from build123d import *

# Parameters (mm, degrees)
SKETCH2_R           = 101.6
SKETCH2_R_2         = 76.2
BOSS_EXTRUDE1_DEPTH = 38.1
FILLET2_R           = 12.7
SHELL1_T            = -6.35


with BuildPart() as part:
    # Sketch2 → Boss-Extrude1 (new, symmetric)
    with BuildSketch(Plane.XY):
        with Locations(Location((0, 0, 0), (0, 0, 180))):
            Circle(SKETCH2_R)
        with Locations(Location((0, 0, 0), (0, 0, 180))):
            Circle(SKETCH2_R_2, mode=Mode.SUBTRACT)
    extrude(amount=BOSS_EXTRUDE1_DEPTH, both=True)

    # Fillet2
    fillet2_edges = [part.edges().sort_by_distance(p)[0] for p in [
        (101.6, 0, -38.1),
        (101.6, 0, 38.1),
    ]]
    fillet(fillet2_edges, radius=FILLET2_R)

    # Shell1
    shell1_openings = [part.faces().sort_by_distance(p)[0] for p in [
        (76.2, 0, 0),
    ]]
    offset(amount=SHELL1_T, openings=shell1_openings, kind=Kind.INTERSECTION)


solid = part.part
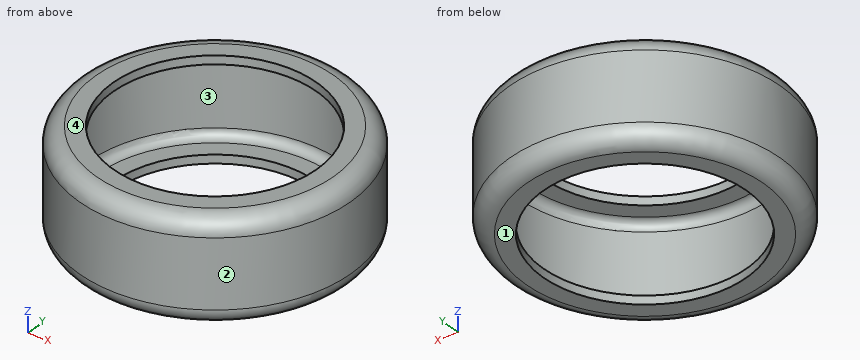
Here's how the part is built. I have some questions about the finished solid (model axes, mm). Face numbers are marked on the shaded views. Round coordinates to 2 decimals unless told otherwise and drop trailing zeros. Loops run counter-clockwise (first coordinate to the right, second up) from the corner with the lowest first, then second, coordinate; pieces in that order, holes last. Notation, with made-up numbers: (-10, -7) - (7, -7) arc R17 ccw to (7, 18) - close; hole circle Ø6 at (2, 65). An arc over 180 degrees is marked (long way). One line per question, with ' | ' between items. Start each with the question number.
Q1. Please list where these lines run through material, in increasing order: line 1 (Z direction, x = 62.5, y = -58); line 2 (Y direction, x = 0, z = 12); line 3 (Z direction, x = -5.5, y = 92.5). Write a range as [from, to].
Q2. Will these pins go through, and if not, where does the flat tip stop? pin 1 (8 mm diameter, centred on y = -68, z = -28, fed in from +X); pin 2 (3 mm diameter, centred on y = -36.5, z = -12, fed in from -X); pin 3 (10 mm diameter, centred on y = -42.5, z = -2.5, fed in from +X).
Q3. I want a section at A-A (y = 0). Write out the boundary of the cut face in (x, z).
Q4. I want a section at C-C (z = -4). Write out the boundary of the cut face in (x, y), then the cut area to 3 significant figures.
Q5. We'd pull the mould along Z, two halves only. Please class the marked faces 1, 2, 3 and 4: +Z half, -Z half, draft (parallel to the pull), parting line (faces both ways), or undercut.
Response values:
1) line 1: z = [-38.1, -31.75], [31.75, 38.1] | line 2: y = [-101.6, -95.25], [95.25, 101.6] | line 3: z = [-37.53, -30.51], [30.51, 37.53]
2) pin 1: stops at x = 78.68 | pin 2: stops at x = -95.38 | pin 3: stops at x = 94.43
3) outline: (-101.6, -25.4) arc R12.7 ccw to (-88.9, -38.1) - (-76.2, -38.1) - (-76.2, -31.75) - (-88.9, -31.75) arc R6.35 cw to (-95.25, -25.4) - (-95.25, 25.4) arc R6.35 cw to (-88.9, 31.75) - (-76.2, 31.75) - (-76.2, 38.1) - (-88.9, 38.1) arc R12.7 ccw to (-101.6, 25.4) - close; (76.2, -38.1) - (88.9, -38.1) arc R12.7 ccw to (101.6, -25.4) - (101.6, 25.4) arc R12.7 ccw to (88.9, 38.1) - (76.2, 38.1) - (76.2, 31.75) - (88.9, 31.75) arc R6.35 cw to (95.25, 25.4) - (95.25, -25.4) arc R6.35 cw to (88.9, -31.75) - (76.2, -31.75) - close
4) outline: circle Ø203.2 at (0, 0); hole circle Ø190.5 at (0, 0) | area: 3,930 mm²
5) face 1: -Z half | face 2: draft | face 3: undercut | face 4: +Z half
